Here's how the part is built. I have some questions about the finished solid (model axes, mm). A direction names the side the tool comes from. Coordinates: 2 decimals unless noted, no trailing zeros. Write each loop counter-clockwise with the first axis right and the second up, starting at its lowest first coordinate (ties: lowest second). Pieces come first, ordered by that corner, then holes.
Item 1: I want a section at C-C (z = 4.5). Please give me the cut outline in (x, y), and give its area (3 significant figures).
Item 2: I want a section at B-B (y = 0). Please give me the cut outline in (x, z).
Item 3: I want a section at D-D (y = 37). Please give me the cut outline in (x, z).
Item 4: I want a section at A-A (x = 0). Please give me the cut outline in (y, z).
Item 5: I'm going to push flat-ended pins straight in: P1, Ø9, axis at x = 32.5, y = 35, coming from the +Z side; P2, Ø6, axis at x = -19, y = 11, coming from the -Z side. Where does each tip first touch, or does it pass through?
Item 6: For faces 1 (the face through (-19, 21, 10)), 2 (the face through (-5.7, -20.5, 3)), 3 (the face through (0, -45, 5)), which set-ups out of +Z, -Z, +X, -X, +Y, -Y let a thin tool reach every point of the face, with its end or its side?
Item 7: If we mould it in two halves opening along Y, with no side actions, what happens to faces 4 (the face through (14, -16, 15)), 5 (the face through (33.021, 38.966, 4.93)), 6 (the face through (-5.85, -26.36, 12.54))? For each: pulls with the +Y half, pulls with the -Y half, needs draft (parallel to the pull), parting line crosses it, or undercut.
Item 8: Please list where these lines run through material, in increasing order: line 1 (Y direction, x = -32.5, z = 4.25); line 2 (Y direction, x = 0, z = 1.5); line 3 (Z direction, x = 8.5, y = -35).
from build123d import *

# Parameters (mm, degrees)
SZKIC1_W                                             = 85
SZKIC1_H                                             = 90
DODANIE_WYCI_GNI_CIE1_DEPTH                          = 10
DODANIE_WYCI_GNI_CIE2_START                          = 5
SZKIC9_R                                             = 27
SZKIC9_R_2                                           = 21
DODANIE_WYCI_GNI_CIE2_DEPTH                          = 5
ZAOKR_GLENIE1_R                                      = 10
POG_BIENIE_STO_KOWE_POD_M6_WKR_T_USTALAJ_D           = 6.4
POG_BIENIE_STO_KOWE_POD_M6_WKR_T_USTALAJ_DEPTH       = 26
POG_BIENIE_STO_KOWE_POD_M6_WKR_T_USTALAJ_CSINK_D     = 13.44
POG_BIENIE_STO_KOWE_POD_M6_WKR_T_USTALAJ_CSINK_ANGLE = 90
POG_BIENIE_STO_KOWE_POD_M6_WKR_T_USTALAJ_TIP         = 1.922753981
SZKIC12_R                                            = 4
WYTNIJ_WYCI_GNI_CIE2_DEPTH                           = 64.688696014


with BuildPart() as part:
    # Szkic1 → Dodanie-wyciągnięcie1 (new body)
    with BuildSketch(Plane.XY):
        Rectangle(SZKIC1_W, SZKIC1_H)
    extrude(amount=DODANIE_WYCI_GNI_CIE1_DEPTH)

    # Szkic2 → Wycięcie-obrót1 (revolve, cut)
    with BuildSketch(Plane(origin=(0, 0, 0), x_dir=(1, 0, 0), z_dir=(0, 1, 0))):
        Polygon((0, 0), (25, 0), (25, -3), (21, -3), (21, -10), (0, -10), align=None)
    revolve(axis=Axis((0, 0, 0), (0, 0, -1)), mode=Mode.SUBTRACT)

    # Szkic9 → Dodanie-wyciągnięcie2 (add)
    with BuildSketch(Plane.XY.offset(10).offset(DODANIE_WYCI_GNI_CIE2_START)):
        Circle(SZKIC9_R)
        Circle(SZKIC9_R_2, mode=Mode.SUBTRACT)
    extrude(amount=-DODANIE_WYCI_GNI_CIE2_DEPTH)

    # Zaokrąglenie1
    zaokr_glenie1_edges = [part.edges().sort_by_distance(p)[0] for p in [
        (42.5, -45, 5),
        (-42.5, -45, 5),
        (-42.5, 45, 5),
        (42.5, 45, 5),
    ]]
    fillet(zaokr_glenie1_edges, radius=ZAOKR_GLENIE1_R)

    # Pogłębienie stożkowe pod M6 Wkręt ustalający1
    with Locations(Plane(origin=(267.5, 155, -16), x_dir=(1, 0, 0), z_dir=(0, 0, -1))):
        with Locations((-235, 190), (-235, 120), (-300, 120), (-300, 190)):
            CounterSinkHole(POG_BIENIE_STO_KOWE_POD_M6_WKR_T_USTALAJ_D / 2, POG_BIENIE_STO_KOWE_POD_M6_WKR_T_USTALAJ_CSINK_D / 2, depth=POG_BIENIE_STO_KOWE_POD_M6_WKR_T_USTALAJ_DEPTH, counter_sink_angle=POG_BIENIE_STO_KOWE_POD_M6_WKR_T_USTALAJ_CSINK_ANGLE)
            with Locations((0, 0, -(POG_BIENIE_STO_KOWE_POD_M6_WKR_T_USTALAJ_DEPTH + POG_BIENIE_STO_KOWE_POD_M6_WKR_T_USTALAJ_TIP / 2))):  # 118° drill point
                Cone(0, POG_BIENIE_STO_KOWE_POD_M6_WKR_T_USTALAJ_D / 2, POG_BIENIE_STO_KOWE_POD_M6_WKR_T_USTALAJ_TIP, mode=Mode.SUBTRACT)

    # Szkic12 → Wytnij-wyciągnięcie2 (cut, through all)
    with BuildSketch(Plane(origin=(0, 0, 0), x_dir=(-1, 0, 0), z_dir=(0, 0, -1))):
        with Locations((-32.5, 35)):
            Circle(SZKIC12_R)
        with Locations((32.5, 35)):
            Circle(SZKIC12_R)
        with Locations((32.5, -35)):
            Circle(SZKIC12_R)
        with Locations((-32.5, -35)):
            Circle(SZKIC12_R)
    extrude(amount=-WYTNIJ_WYCI_GNI_CIE2_DEPTH, mode=Mode.SUBTRACT)


solid = part.part
Answer:
1. outline: (-42.5, -35) arc R10 ccw to (-32.5, -45) - (32.5, -45) arc R10 ccw to (42.5, -35) - (42.5, 35) arc R10 ccw to (32.5, 45) - (-32.5, 45) arc R10 ccw to (-42.5, 35) - close; hole circle Ø8 at (-32.5, -35); hole circle Ø8 at (-32.5, 35); hole circle Ø42 at (0, 0); hole circle Ø8 at (32.5, -35); hole circle Ø8 at (32.5, 35)
1. area: 5,980 mm2
2. outline: (-42.5, 0) - (-25, 0) - (-25, 3) - (-21, 3) - (-21, 15) - (-27, 15) - (-27, 10) - (-42.5, 10) - close; (21, 3) - (25, 3) - (25, 0) - (42.5, 0) - (42.5, 10) - (27, 10) - (27, 15) - (21, 15) - close
3. outline: (-42.3, 0) - (-35.96, 0) - (-35.96, 10) - (-42.3, 10) - close; (-29.04, 0) - (29.04, 0) - (29.04, 10) - (-29.04, 10) - close; (35.96, 0) - (42.3, 0) - (42.3, 10) - (35.96, 10) - close
4. outline: (-45, 0) - (-25, 0) - (-25, 3) - (-21, 3) - (-21, 15) - (-27, 15) - (-27, 10) - (-45, 10) - close; (21, 3) - (25, 3) - (25, 0) - (45, 0) - (45, 10) - (27, 10) - (27, 15) - (21, 15) - close
5. P1: stops at z = 10
5. P2: stops at z = 3
6. face 1: +Z
6. face 2: -Z
6. face 3: +Z, -Z, +X, -X, -Y
7. face 4: needs draft
7. face 5: undercut
7. face 6: parting line crosses it
8. line 1: y = -45 to -39, -31 to 31, 39 to 45
8. line 2: y = -45 to -25, 25 to 45
8. line 3: z = 0 to 10
